Check sheet for the modelled part. Datum: model origin and axes. Units: mm. Face numbers are marked on the shaded views. Round coordinates to 2 decimals unless told otherwise and drop trailing zeros. Write each loop counter-clockwise with the first axis right and the second up, starting at its lowest first coordinate (ties: lowest second). Pieces come first, ordered by that corner, then holes.
Item 1: Release check for a two-part mould opening along Y. For the marked faces 1, 2 and 3 record: pulls with the +Y half, pulls with the -Y half, needs draft (parallel to the pull), parting line crosses it, or undercut.
Item 2: Material ranges on line 1 along Y through (x, z) = (1.2, 2.3); line 2 along Z through (x, y) = (3.75, -8); line 3 along Y through (x, z) = (1.8, 0.4), recorded low to high.
Item 3: Section check B-B, the plane y = -20.7. Record the cut outline in (x, z), plus the area to 3 significant figures.
Item 4: Section check C-C, the plane y = -8.5. Record the cut outline in (x, z), plus the area to 3 significant figures.
Item 5: Section check D-D, the plane x = 1.2. State how many separate pieces and enclosed holes the cut face has, plus the area to 3 significant figures.
Item 6: Depth check by flat-ended pin: pin 1 (6 mm diameter, centred on x = 14, y = -7, fed in from -Z); pin 2 (0.8 mm diameter, centred on x = 3, z = 2, fed in from -Y); pin 3 (0.8 mm diameter, centred on x = 3.5, z = 3, fed in from +Y); pin 4 (1.5 mm diameter, centred on x = 10.5, z = 3, fed in from -Y). Enter the tip coordinate at first touch or a pass-through.
Item 7: Section check A-A, the plane y = -12.55. Record the cut outline in (x, z), plus the area to 4 significant figures.
from build123d import *

# Parameters (mm, degrees)
SALIENTE_EXTRUIR1_DEPTH    = 5
CROQUIS3_R                 = 1
CORTAR_EXTRUIR1_DEPTH      = 5
REDONDEO2_R                = 2.5
CROQUIS4_W                 = 2.5
CROQUIS4_H                 = 9.3
CORTAR_EXTRUIR2_DEPTH      = 4.8
CORTAR_EXTRUIR3_DEPTH      = 37.123740235
CORTAR_EXTRUIR3_DEPTH_BACK = 37.123740235
CROQUIS5_R                 = 1


with BuildPart() as part:
    # Croquis2 → Saliente-Extruir1 (new body)
    with BuildSketch(Plane.XY):
        with BuildLine():
            Line((0, 0), (0, -25))
            add(Edge.make_bspline(
                [(0, -25), (12.595125448, -26.182989262), (25, -25)],
                knots=[0, 0, 0, 0.592275768, 0.592275768, 0.592275768], degree=2))
            Line((25, -25), (0, 0))
        make_face()
    extrude(amount=SALIENTE_EXTRUIR1_DEPTH)

    # Croquis3 → Cortar-Extruir1 (cut)
    with BuildSketch(Plane.XY.offset(5)):
        with Locations((1.2, -20.7)):
            Circle(CROQUIS3_R)
    extrude(amount=-CORTAR_EXTRUIR1_DEPTH, mode=Mode.SUBTRACT)

    # Redondeo2
    redondeo2_edges = [part.edges().sort_by_distance(p)[0] for p in [
        (0, -25, 2.5),
    ]]
    fillet(redondeo2_edges, radius=REDONDEO2_R)

    # Croquis4 → Cortar-Extruir2 (cut)
    with BuildSketch(Plane.ZY):
        with Locations((2.501199275, -12.55)):
            Rectangle(CROQUIS4_W, CROQUIS4_H)
    extrude(amount=-CORTAR_EXTRUIR2_DEPTH, mode=Mode.SUBTRACT)

    # Croquis5 → Cortar-Extruir3 (cut, two sides: drawn at the far end of the back side and taken through both)
    with BuildSketch(Plane.XY.offset(5).offset(-CORTAR_EXTRUIR3_DEPTH_BACK)):
        with Locations(Location((1.8, -12.55, 0), (0, 0, 270))):
            Circle(CROQUIS5_R)
    extrude(amount=CORTAR_EXTRUIR3_DEPTH + CORTAR_EXTRUIR3_DEPTH_BACK, mode=Mode.SUBTRACT)


solid = part.part
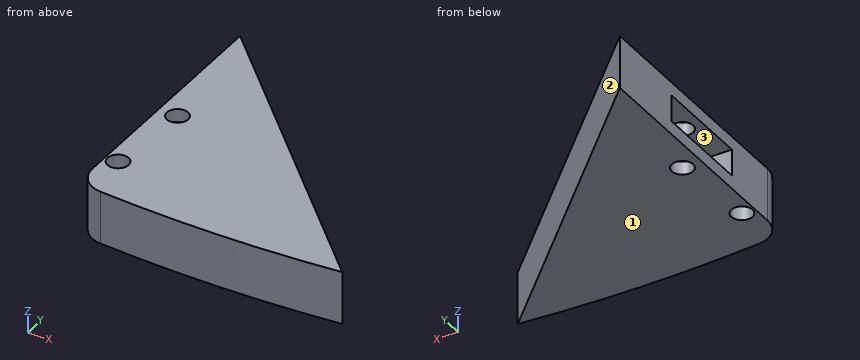
Values found:
1. face 1: needs draft
1. face 2: pulls with the +Y half
1. face 3: undercut
2. line 1: y = -24.84 to -21.7, -19.7 to -17.2, -7.9 to -1.2
2. line 2: z = 0 to 1.25, 3.75 to 5
2. line 3: y = -25.1 to -21.5, -19.9 to -13.55, -11.55 to -1.8
3. outline: (0, 0) - (0.2, 0) - (0.2, 5) - (0, 5) - close; (2.2, 0) - (20.7, 0) - (20.7, 5) - (2.2, 5) - close
3. area: 93.5 mm2
4. outline: (0, 0) - (8.5, 0) - (8.5, 5) - (0, 5) - (0, 3.75) - (4.8, 3.75) - (4.8, 1.25) - (0, 1.25) - close
4. area: 30.5 mm2
5. separate pieces: 3
5. enclosed holes: 0
5. area: 80.9 mm2
6. pin 1: passes through
6. pin 2: stops at y = -25.28
6. pin 3: stops at y = -3.1
6. pin 4: stops at y = -25.59
7. outline: (0, 0) - (0.8, 0) - (0.8, 1.25) - (0, 1.25) - close; (0, 3.75) - (0.8, 3.75) - (0.8, 5) - (0, 5) - close; (2.8, 0) - (12.55, 0) - (12.55, 5) - (2.8, 5) - (2.8, 3.75) - (4.8, 3.75) - (4.8, 1.25) - (2.8, 1.25) - close
7. area: 45.75 mm2
